Could you check a few things on this model? Use its own coordinates, in mm. Round coordinates to 2 decimals unless told otherwise and drop trailing zeros. Write each loop counter-clockwise with the first axis right and the second up, starting at its lowest first coordinate (ties: lowest second). Pieces come first, ordered by that corner, then holes. Notation, with made-up numbers: (48.5, 76.25) -> (95.5, 76.25) arc R33 ccw to (95.5, 110.25) -> close; hole circle Ø2 at (7.25, 86). An arc over 180 degrees is marked (long way). Return JSON: item names as keys, results as strings.
from build123d import *

# Parameters (mm, degrees)
F0_W     = 762
F0_H     = 711.2
F1_DEPTH = 19.05
F3_DEPTH = 25.4


with BuildPart() as f1:
    # F0 (on Right) → F1 (new body)
    with BuildSketch(Plane.YZ):
        Rectangle(F0_W, F0_H)
    extrude(amount=F1_DEPTH)

    # F2 (on face) → F3 (cut)
    with BuildSketch(Plane.YZ.offset(19.05)):
        with BuildLine():
            ThreePointArc((-44.45, 355.6), (0, 311.15), (44.45, 355.6))
            Line((44.45, 355.6), (-44.45, 355.6))
        make_face()
    extrude(amount=-F3_DEPTH, mode=Mode.SUBTRACT)


solid = f1.part
1) Thinking about a two-plate mould opening in Y: for faces 1 (the face through (9.66, -0.98, 311.16)), 2 (the face through (9, 381, -5)), 3 (the face through (9, -5, -355.6)), which applies, pulls with the +Y half, pulls with the -Y half, needs draft (parallel to the pull), parting line crosses it, or undercut?
Return value:
{"face 1": "undercut", "face 2": "pulls with the +Y half", "face 3": "needs draft"}
2) I want a section at A-A, the plane y = 0. Please give me the cut outline in (x, z).
Return value:
{"outline": "(0, -355.6) -> (19.05, -355.6) -> (19.05, 311.15) -> (0, 311.15) -> close"}
3) If I drill on probe 1 along Z at (x, y) = (6.5, -5.5); probe 2 along Z at (x, y) = (12, -27.5), over which ranges is the centre line in solid material (lowest first)? Write a range as [from, to].
Return value:
{"probe 1": "[-355.6, 311.49]", "probe 2": "[-355.6, 320.68]"}
4) Will this pin go through, and if not, where does the flat tip stop? pin 1 Ø4 at (x, y) = (3, -19.5) entering from +Z.
Return value:
{"pin 1": "z = 316.7"}
